Read the model definition and answer for the solid it produces. Units are mm, in the model's axes. Face numbers are marked on the shaded views. A direction names the side the tool comes from. Round coordinates to 2 decimals unless told otherwise and drop trailing zeros. Write each loop counter-clockwise with the first axis right and the second up, starting at its lowest first coordinate (ties: lowest second). Pieces come first, ordered by that corner, then holes.
Autodesk Inventor part; units mm, degrees
ref_plane "YZ Plane" through (0, 0, 0) normal (1, 0, 0) x (0, 1, 0)
ref_plane "XZ Plane" through (0, 0, 0) normal (0, 1, 0) x (-1, 0, 0)
ref_plane "XY Plane" through (0, 0, 0) normal (0, 0, 1) x (1, 0, 0)
sketch "スケッチ1" plane through (0, 0, 0) normal (0, 0, 1) x (1, 0, 0)
  line L0 (0, 0) -> (38, 0)
  line L1 (38, 0) -> (38, 24)
  line L2 (38, 24) -> (0, 24)
  line L3 (0, 24) -> (0, 0)
  line L4 (0, 4) -> (38, 4)
  line L5 (12.4, 31) -> (25.6, 31)
  line L6 (25.6, 31) -> (25.6, 17)
  line L7 (25.6, 17) -> (12.4, 17)
  line L8 (12.4, 17) -> (12.4, 31)
  arc A0 (25.6, 31) -> (12.4, 31) centre (19, 31) ccw
  arc A1 (12.4, 17) -> (25.6, 17) centre (19, 17) ccw
  line L9 (0, 24) -> (38, 24)
  line L10 (38, 24) -> (38, 44)
  line L11 (38, 44) -> (0, 44)
  line L12 (0, 44) -> (0, 24)
  line L13 (0, 44) -> (38, 44)
  line L14 (38, 44) -> (38, 50)
  line L15 (38, 50) -> (0, 50)
  line L16 (0, 50) -> (0, 44)
  point P0 (19, 24)
  point P1 (19, 39.6)
  point P2 (25.6, 24)
  point P3 (12.4, 24)
  dimension "d0" = 38
  dimension "d1" = 24
  dimension "d2" = 4
  dimension "d3" = 15.6
  dimension "d4" = 13.2
  dimension "d5" = 14
  dimension "d6" = 7
  dimension "d7" = 19
  dimension "d49" = 6
  dimension "d50" = 38
  dimension "d51" = 20
  dimension "d52" = 38
extrude "押し出し1" add sketch "スケッチ1" against normal blind 6 contours L3 L4 L1 L0 | L3 L2 L8 A1 L6 L1 L4 | L12 L11 L10 L2 L6 A0 L8 | L16 L15 L14 L11
extrude "押し出し2" add sketch "スケッチ1" against normal blind 50 contours L3 L4 L1 L0 | L16 L15 L14 L11
sketch "スケッチ2" plane through (0, 0, 0) normal (0, 0, 1) x (1, 0, 0)
  line L0 (0, 50) -> (0, 0)
  line L1 (38, 50) -> (0, 50)
  point P0 (3.5, 25)
  point P1 (19, 25)
  point P2 (11.25, 11.5766)
  point P3 (26.75, 11.5766)
  point P4 (34.5, 25)
  point P5 (26.75, 38.4234)
  point P6 (11.25, 38.4234)
  point P7 (0, 25)
  point P8 (19, 43.6)
  point P9 (0, 25)
  point P10 (19, 50)
  dimension "d16" = 360
  dimension "d18" = 15.5
hole "穴1" at (3.5, 25, 0) at (19, 25, 0) at (11.25, 11.5766, 0) at (26.75, 11.5766, 0) at (34.5, 25, 0) at (26.75, 38.4234, 0) at (11.25, 38.4234, 0) direction (0, 0, -1) diameter 3.3 depth 8.1 tip angle 118
sketch "スケッチ4" plane through (0, 4, -6) normal (0, 1, 0) x (1, 0, 0)
  point P0 (0, -6)
  point P1 (3.1531, 2.3812)
  point P2 (35.1531, 2.3812)
  point P3 (35.1531, 28.3812)
  point P4 (3.1531, 28.3812)
  dimension "d47" = 32
  dimension "d48" = 26
hole "穴3" at (3.1531, 4, -8.3812) at (35.1531, 4, -8.3812) at (35.1531, 4, -34.3812) at (3.1531, 4, -34.3812) direction (0, -1, 0) diameter 3.2 depth 8.1 tip angle 118
equation "\"d51\" = d1 - d2"
properties part number "ギアボックス"
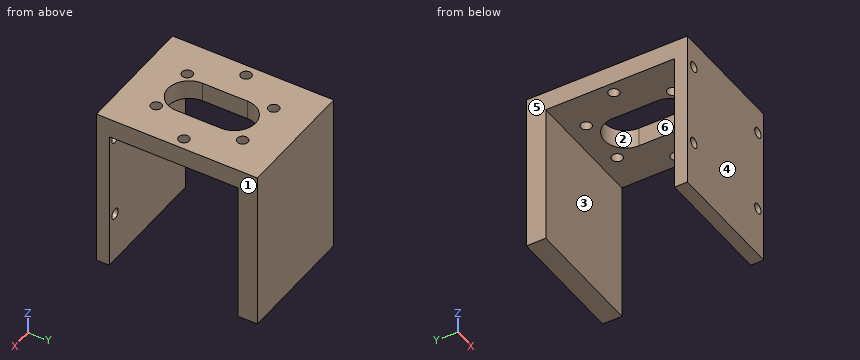
Q1. Flat-ended cylindrical pins translate along their axes: pin 1 Ø1.9 at (x, z) = (3.15, -34.38) entering from -Y; pin 2 Ø4.5 at (x, y) = (11.25, 11.58) entering from -Z. Find the tip coordinate at first contact, or state that the pin passes through.
Verdict:
pin 1: stops at y = 44
pin 2: stops at z = -6
Q2. Determine the mould class of the marked faces 4, 5 and 6 for opening direction Y: pulls with the +Y half, pulls with the -Y half, needs draft (parallel to the pull), parting line crosses it, or undercut.
Verdict:
face 4: pulls with the -Y half
face 5: needs draft
face 6: undercut
Q3. Section D-D (z = -17) is taken. Determine the outline of the cut face in (x, y).
Verdict:
outline: (0, 0) - (38, 0) - (38, 4) - (0, 4) - close; (0, 44) - (38, 44) - (38, 50) - (0, 50) - close
Q4. Section B-B (y = 25) is taken. Determine the outline of the cut face in (x, z).
Verdict:
outline: (0, -6) - (1.85, -6) - (1.85, 0) - (0, 0) - close; (5.15, -6) - (12.4, -6) - (12.4, 0) - (5.15, 0) - close; (25.6, -6) - (32.85, -6) - (32.85, 0) - (25.6, 0) - close; (36.15, -6) - (38, -6) - (38, 0) - (36.15, 0) - close
Q5. Section A-A (x = 26.75) is taken. Determine the outline of the cut face in (y, z).
Verdict:
outline: (0, -50) - (4, -50) - (4, -6) - (9.93, -6) - (9.93, 0) - (0, 0) - close; (13.23, -6) - (36.77, -6) - (36.77, 0) - (13.23, 0) - close; (40.07, -6) - (44, -6) - (44, -50) - (50, -50) - (50, 0) - (40.07, 0) - close
Q6. Which of the six approach directions +Z, -Z, +X, -X, +Y, -Y give full straight-line access (tool end or side, diameter ignored) to the marked faces 1, 2 and 3?
Verdict:
face 1: +Z, -Z, +X, +Y, -Y
face 2: +Z, -Z
face 3: -Z, +X, -X
Q7. Straight lines are drawn through the part: probe 1 along Y at (x, z) = (11.25, -2.1); probe 2 along Y at (x, z) = (29, -27); probe 3 along Y at (x, z) = (26, -1). For each, find the intervals that lie inside material, in ascending order.
Verdict:
probe 1: y = 0 to 9.93, 13.23 to 36.77, 40.07 to 50
probe 2: y = 0 to 4, 44 to 50
probe 3: y = 0 to 10.11, 13.05 to 36.95, 39.89 to 50
Q8. Section C-C (x = 19) is taken. Determine the outline of the cut face in (y, z), then the cut area to 3 significant figures.
Verdict:
outline: (0, -50) - (4, -50) - (4, -6) - (10.4, -6) - (10.4, 0) - (0, 0) - close; (37.6, -6) - (44, -6) - (44, -50) - (50, -50) - (50, 0) - (37.6, 0) - close
area: 577 mm2
